from build123d import *

# Parameters (mm, degrees)
SALIENTE_EXTRUIR1_DEPTH = 3


with BuildPart() as part:
    # Croquis1 → Saliente-Extruir1 (new body)
    with BuildSketch(Plane(origin=(0, 0, 0), x_dir=(0, 0, -1), z_dir=(1, 0, 0))):
        with BuildLine():
            Line((24.5, 167), (70.5, 167))
            Line((70.5, 167), (70.5, 170))
            Line((70.5, 170), (95, 170))
            Line((95, 170), (95, 108))
            Line((95, 108), (92, 108))
            Line((92, 108), (92, 62))
            Line((92, 62), (95, 62))
            Line((95, 62), (95, 0))
            Line((95, 0), (70.5, 0))
            Line((70.5, 0), (70.5, 3))
            Line((70.5, 3), (50.5, 3))
            Line((50.5, 3), (50.5, 6))
            ThreePointArc((50.5, 6), (47.5, 9), (44.5, 6))
            Line((44.5, 6), (44.5, 3))
            Line((44.5, 3), (24.5, 3))
            Line((24.5, 3), (24.5, 0))
            Line((24.5, 0), (0, 0))
            Line((0, 0), (0, 62))
            Line((0, 62), (3, 62))
            Line((3, 62), (3, 108))
            Line((3, 108), (0, 108))
            Line((0, 108), (0, 170))
            Line((0, 170), (24.5, 170))
            Line((24.5, 170), (24.5, 167))
        make_face()
    extrude(amount=SALIENTE_EXTRUIR1_DEPTH)


solid = part.part
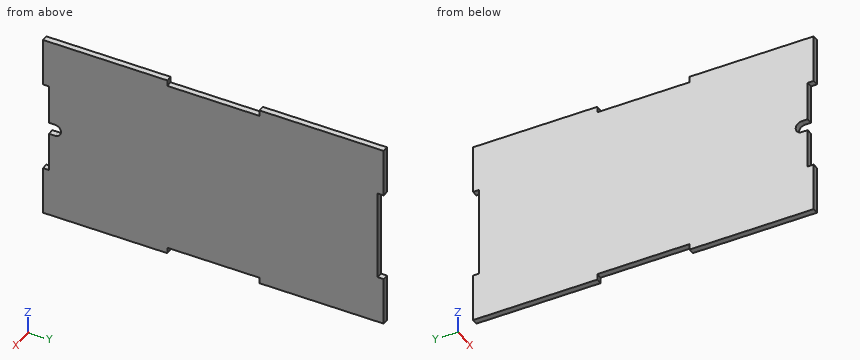
The model under review builds one solid part; all positions refer to its coordinate system, in mm. Coordinates: 2 decimals unless noted, no trailing zeros. Loops run counter-clockwise (first coordinate to the right, second up) from the corner with the lowest first, then second, coordinate; pieces in that order, holes last.
(1) Consider section B-B, the plane z = -47.5. Give the boundary of the cut face in (x, y), plus the area to 3 significant figures.
Determined:
outline: (0, 9) - (3, 9) - (3, 167) - (0, 167) - close
area: 474 mm2
(2) Insertion check: P1, Ø3, axis at y = 34, z = -57, coming from the -X side; P2, Ø1.5, axis at x = 1.5, z = -65, coming from the -Y side; P3, Ø0.9, axis at x = 2, y = 77, coming from the -Z side. Each pin has a flat end and moves straight along its axis. Give the tip position at first contact, or say it passes through.
Determined:
P1: stops at x = 0
P2: stops at y = 3
P3: stops at z = -92
(3) Wall thickness on L1, parallel to Y at x = 2.7, z = -58; L2, parallel to Z at x = 0.55, y = 95.5; L3, parallel to Z at x = 1.25, y = 8.5: over which ranges is each line inside the solid? List them lowest first.
Determined:
L1: y = 3 to 167
L2: z = -92 to -3
L3: z = -95 to -49.16, -45.84 to 0
(4) Consider section A-A, the plane x = 1.6. Give the boundary of the cut face in (y, z).
Determined:
outline: (0, -95) - (62, -95) - (62, -92) - (108, -92) - (108, -95) - (170, -95) - (170, -70.5) - (167, -70.5) - (167, -24.5) - (170, -24.5) - (170, 0) - (108, 0) - (108, -3) - (62, -3) - (62, 0) - (0, 0) - (0, -24.5) - (3, -24.5) - (3, -44.5) - (6, -44.5) arc R3 cw to (6, -50.5) - (3, -50.5) - (3, -70.5) - (0, -70.5) - close
(5) Consider section C-C, the plane z = -28. Give the boundary of the cut face in (x, y), plus the area to 3 significant figures.
Determined:
outline: (0, 3) - (3, 3) - (3, 167) - (0, 167) - close
area: 492 mm2
